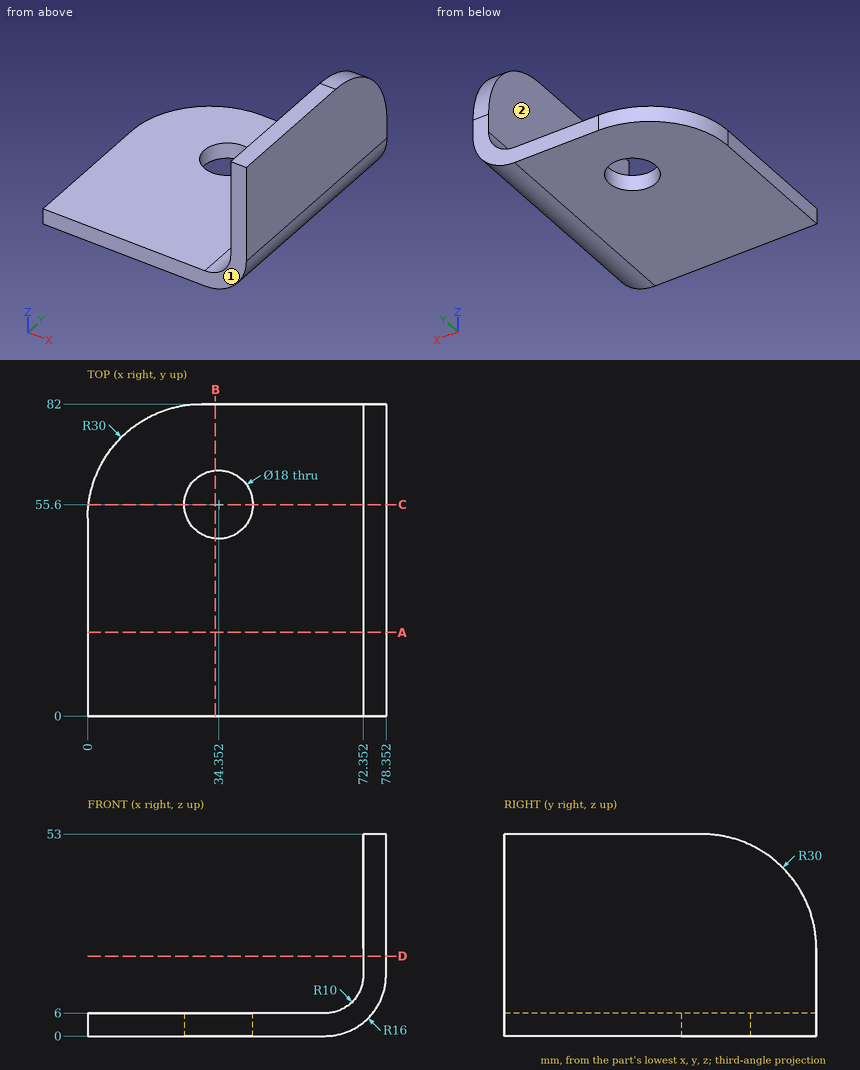
Verification items for this drawing (mm, ordinates from the low corner). A direction names the side the tool comes from. Coordinates: 2 decimals unless noted, no trailing zeros. Order: outer loops, then holes, each group sorted by start corner. A loop starts at its lowest first (then second) coordinate and runs counter-clockwise, first axis right, second up. Notation, with made-up numbers: (1.5, 34.25) - (7.5, 34.25) arc R16 ccw to (7.5, 40.25) - close; hole circle Ø8 at (-1, 55). An arc over 180 degrees is marked (long way). Answer in a Markdown table with one row per item. Add a question column.
1. Material ranges on L1, parallel to Z at x = 49, y = 69; L2, parallel to X at y = 42, z = 20; L3, parallel to X at y = 55.6, z = 2.5 (1 decimal), recorded low to high. Write a range as [from, to].
2. Gauge pin test, flat ends, axial feed: pin 1 Ø5 at (x, y) = (66.5, 69.5) entering from +Z; pin 2 Ø2 at (y, z) = (17, 13) entering from +X; pin 3 Ø10 at (y, z) = (60.5, 9.5) entering from +X. Record the tip position at first contact, or that the pin passes through.
3. Section check B-B (x = 33.5). Enter the section's corners in (y, z).
4. Access from +Z, -Z, +X, -X, +Y, -Y to the whole of each face (thin tool, end or side, straight path). Record for the marked faces 1 and 2.
5. Section check C-C (y = 55.6). Enter the section's corners in (x, z).
6. Section check D-D (z = 21). Enter the section's corners in (x, y).
7. Section check A-A (y = 22). Enter the section's corners in (x, z), plus the area to 3 significant figures.
Data:
| question | item | result |
|---|---|---|
| 1 | L1 | z = [0, 6] |
| 1 | L2 | x = [72.35, 78.35] |
| 1 | L3 | x = [0.2, 25.4], [43.4, 70.9] |
| 2 | pin 1 | stops at z = 8.53 |
| 2 | pin 2 | stops at x = 78.23 |
| 2 | pin 3 | stops at x = 78.28 |
| 3 | outline | (0, 0) - (46.64, 0) - (46.64, 6) - (0, 6) - close; (64.56, 0) - (82, 0) - (82, 6) - (64.56, 6) - close |
| 4 | face 1 | +Z, -Z, +X, -X, -Y |
| 4 | face 2 | +Z, -X, +Y, -Y |
| 5 | outline | (0.22, 0) - (25.35, 0) - (25.35, 6) - (0.22, 6) - close; (43.35, 0) - (62.35, 0) arc R16 ccw to (78.35, 16) - (78.35, 52.78) - (72.35, 52.78) - (72.35, 16) arc R10 cw to (62.35, 6) - (43.35, 6) - close |
| 6 | outline | (72.35, 0) - (78.35, 0) - (78.35, 82) - (72.35, 82) - close |
| 7 | outline | (0, 0) - (62.35, 0) arc R16 ccw to (78.35, 16) - (78.35, 53) - (72.35, 53) - (72.35, 16) arc R10 cw to (62.35, 6) - (0, 6) - close |
| 7 | area | 719 mm² |
